CAD build for the part. Positions are in the model's coordinates, mm. A direction names the side the tool comes from. Coordinates: 2 decimals unless noted, no trailing zeros. Loops run counter-clockwise (first coordinate to the right, second up) from the corner with the lowest first, then second, coordinate; pieces in that order, holes last. Notation, with made-up numbers: (59, 30.25) -> (110, 30.25) arc R14 ccw to (110, 55.25) -> close; hole circle Ø8 at (42, 32.5). An arc over 180 degrees is marked (long way). Write each question's results on one line, items separated by ' | '.
```python
from build123d import *

# Parameters (mm, degrees)
SKETCH4_R                = 6.35
CUT_EXTRUDE1_DEPTH       = 100.595858348
RIB9_REACH               = 103.996
SKETCH6_WALL_W           = 233.119417624
SKETCH6_WALL_H           = 3.175
FILLET1_R                = 1.5875
CIRPATTERN1_COUNT        = 8
FILLET1_OF_CIRPATTERN1_R = 1.5875


with BuildPart() as part:
    # Sketch3 → Revolve1 (revolve)
    with BuildSketch(Plane.XY, mode=Mode.PRIVATE) as revolve1_sk:
        Polygon((0, 25.4), (9.525, 25.4), (12.7, 22.225), (12.7, 12.7), (69.85, 12.7), (69.85, 0), (0, 0), align=None)
    revolve(revolve1_sk.sketch.rotate(Axis((0, 0, 0), (0, 1, 0)), 90), axis=Axis((0, 0, 0), (0, 1, 0)))

    # Sketch4 → Cut-Extrude1 (cut, through all)
    with BuildSketch(Plane(origin=(0, 12.7, 0), x_dir=(1, 0, 0), z_dir=(0, 1, 0))):
        with Locations(Location((0, 55.5625, 0), (0, 0, 270))):
            Circle(SKETCH4_R)
        with Locations(Location((24.107665255, 50.060082723, 0), (0, 0, 270))):
            Circle(SKETCH4_R)
        with Locations(Location((43.440511745, 34.642652116, 0), (0, 0, 270))):
            Circle(SKETCH4_R)
        with Locations(Location((54.169432121, 12.363819393, 0), (0, 0, 270))):
            Circle(SKETCH4_R)
        with Locations(Location((54.169432121, -12.363819393, 0), (0, 0, 270))):
            Circle(SKETCH4_R)
        with Locations(Location((43.440511745, -34.642652116, 0), (0, 0, 270))):
            Circle(SKETCH4_R)
        with Locations(Location((24.107665255, -50.060082723, 0), (0, 0, 270))):
            Circle(SKETCH4_R)
        with Locations(Location((0, -55.5625, 0), (0, 0, 270))):
            Circle(SKETCH4_R)
        with Locations(Location((-24.107665255, -50.060082723, 0), (0, 0, 270))):
            Circle(SKETCH4_R)
        with Locations(Location((-43.440511745, -34.642652116, 0), (0, 0, 270))):
            Circle(SKETCH4_R)
        with Locations(Location((-54.169432121, -12.363819393, 0), (0, 0, 270))):
            Circle(SKETCH4_R)
        with Locations(Location((-54.169432121, 12.363819393, 0), (0, 0, 270))):
            Circle(SKETCH4_R)
        with Locations(Location((-43.440511745, 34.642652116, 0), (0, 0, 270))):
            Circle(SKETCH4_R)
        with Locations(Location((-24.107665255, 50.060082723, 0), (0, 0, 270))):
            Circle(SKETCH4_R)
    extrude(amount=-CUT_EXTRUDE1_DEPTH, mode=Mode.SUBTRACT)

    # Sketch6 wall → Rib9 (add, up to next)
    with BuildSketch(Plane(origin=(0, 17.4625, -25.4), x_dir=(0, -0.351123441588, -0.936329177569), z_dir=(0, 0.936329177569, -0.351123441588)), mode=Mode.PRIVATE) as rib9_sk1:
        Rectangle(SKETCH6_WALL_W, SKETCH6_WALL_H)
    rib9_tool1 = extrude(rib9_sk1.sketch, amount=-RIB9_REACH, mode=Mode.PRIVATE) - part.part
    rib9 = rib9_tool1.solids().sort_by_distance((0, 17.4625, -25.4))[0]
    add(rib9)

    # Fillet1
    fillet1_edges = [part.edges().sort_by_distance(p)[0] for p in [
        (1.5875, 12.7, -25.350195309),
        (-1.5875, 12.7, -25.350195309),
    ]]
    fillet(fillet1_edges, radius=FILLET1_R)

    # CirPattern1: Rib9 ×8 about axis
    cirpattern1_axis = Axis((0, 0, 0), (0, 1, 0))
    for i in range(1, CIRPATTERN1_COUNT):
        add(rib9.rotate(cirpattern1_axis, i * 360 / CIRPATTERN1_COUNT))

    # Fillet1 of CirPattern1
    fillet1_of_cirpattern1_edges = [part.edges().sort_by_distance(p)[0] for p in [
        (-16.802762993, 12.7, -19.047827023),
        (-19.047827023, 12.7, -16.802762993),
        (-25.350195309, 12.7, -1.5875),
        (-25.350195309, 12.7, 1.5875),
        (-19.047827023, 12.7, 16.802762993),
        (-16.802762993, 12.7, 19.047827023),
        (-1.5875, 12.7, 25.350195309),
        (1.5875, 12.7, 25.350195309),
        (16.802762993, 12.7, 19.047827023),
        (19.047827023, 12.7, 16.802762993),
        (25.350195309, 12.7, 1.5875),
        (25.350195309, 12.7, -1.5875),
        (19.047827023, 12.7, -16.802762993),
        (16.802762993, 12.7, -19.047827023),
    ]]
    fillet(fillet1_of_cirpattern1_edges, radius=FILLET1_OF_CIRPATTERN1_R)


solid = part.part
```
Q1. Drop flat-ended pins along their axis: pin 1 (5 mm diameter, centred on x = 10.5, z = -8.5, fed in from -Y); pin 2 (4 mm diameter, centred on y = 18, z = 27.5, fed in from -X); pin 3 (9 mm diameter, centred on y = 17, z = 25.5, fed in from +X); pin 4 (20.5 mm diameter, centred on x = -54.17, z = 12.36, fed in from +Y). Give the stop position or say it passes through.
Results are:
pin 1: y = 0 | pin 2: x = -1.59 | pin 3: x = 65.53 | pin 4: y = 12.7
Q2. Pull direction X, two halves, no side cores. Call faces 1 (the flat face through (-25.14, 17.56, 0.04)), 2 (the flat face through (17.75, 17.56, -17.81)), 3 (the cylindrical face through (-19.816, 6.439, -54.74)): +X half, -X half, draft (parallel to the pull), parting line (faces both ways), or undercut.
Results are:
face 1: -X half | face 2: +X half | face 3: undercut
Q3. Which spindle directions (+Z, -Z, +X, -X, +Y, -Y) get a long thin tool onto all of the face, cutting with end or side? Do faces 4 (the flat face through (20, 17, 1.588)), 5 (the cylindrical face through (16.486, 13.153, 19.406)), 6 (the cylindrical face through (-49.074, 6.439, 37.573)), 7 (the flat face through (1.588, 17, -20)), 8 (the cylindrical face through (-11.715, 17.396, -4.904)). Say none if no direction does.
Results are:
face 4: +X, +Y | face 5: +Z, +Y | face 6: +Y, -Y | face 7: -Z, +Y | face 8: -X, +Y
Q4. Cut at B-B on y = 7. Give the number of separate pieces and of enclosed holes in the cut face, and give its area (3 significant figures).
Results are:
separate pieces: 1 | enclosed holes: 14 | area: 13,600 mm^2
Q5. Wall check: L1, parallel to X at y = 5, z = 37; L2, parallel to X at y = 17.75, z = -13; L3, parallel to Y at x = -15, z = 29.5. Give the ranges that are in metal, low to high. Write a range as from..to.
Results are:
L1: -59.25..-49.34, -37.54..37.54, 49.34..59.25 | L2: -15.25..-10.75, -1.59..1.59, 10.75..15.25 | L3: 0..12.7
Q6. Cut at A-A on z = 36. Write the cut outline in (x, y) (1 decimal), and give its area (3 significant figures).
Results are:
outline: (-59.9, 0) -> (-49.6, 0) -> (-49.6, 12.7) -> (-59.9, 12.7) -> close; (-37.2, 0) -> (37.2, 0) -> (37.2, 12.7) -> (3.2, 12.7) arc R1.6 cw to (1.8, 13.5) -> (-1.8, 13.5) arc R1.6 cw to (-3.2, 12.7) -> (-37.2, 12.7) -> close; (49.6, 0) -> (59.9, 0) -> (59.9, 12.7) -> (49.6, 12.7) -> close | area: 1,210 mm^2
